Source: CAD feature listing. Evaluate the final solid. Frame: model axes, mm. Round coordinates to 2 decimals unless told otherwise and drop trailing zeros. Loops run counter-clockwise (first coordinate to the right, second up) from the corner with the lowest first, then second, coordinate; pieces in that order, holes last. Notation, with made-up numbers: (19.25, 5) -> (35.25, 5) arc R6 cw to (35.25, 15) -> close; hole circle Ø2 at (-31.75, 67). An arc over 180 degrees is marked (long way). Put each result on its own line as item: value. Start each with the question number.
1. Contact query for flat-ended pins moving along their axis: pin 1 (1.6 mm diameter, centred on x = -2, z = 1.5, fed in from +Y); pin 2 (2.5 mm diameter, centred on x = 13, y = -37.25, fed in from -Z); pin 3 (1 mm diameter, centred on y = -40.5, z = 0.5, fed in from +X); pin 4 (1.2 mm diameter, centred on x = -13, y = 37.25, fed in from -Z). Output: stop coordinate, or through.
2. Cut plane A-A (y = 19.5). Return the cut outline in (x, z), then the cut area to 3 significant figures.
3. Material intervals for L1, parallel to Y at x = -2.5, z = 1.2; L2, parallel to Y at x = -1, z = 0.05; L3, parallel to X at y = 10, z = 0.6, sorted ascending.
4. Cut plane D-D (y = -37.25). Return the cut outline in (x, z), then the cut area to 3 significant figures.
5. Cut plane C-C (x = -13). Return the cut outline in (y, z), then the cut area to 3 significant figures.
6. Cut plane B-B (z = 1.25). Return the cut outline in (x, y), then the cut area to 3 significant figures.
```python
from build123d import *

# Parameters (mm, degrees)
F1_DEPTH = 2
F2_R     = 1
F3_DEPTH = 2.001
F4_W     = 11.5
F4_H     = 56.5
F4_H_2   = 6.5
F5_DEPTH = 2.001
F6_W     = 15
F6_H     = 15
F7_DEPTH = 3
F8_SIZE  = 2


with BuildPart() as f1:
    # F0 (on Top) → F1 (new body)
    with BuildSketch(Plane.XY):
        with BuildLine():
            Line((16.75, -33), (16.75, 33))
            ThreePointArc((16.75, 33), (11.844039, 44.844039), (0, 49.75))
            ThreePointArc((0, 49.75), (-11.844039, 44.844039), (-16.75, 33))
            Line((-16.75, 33), (-16.75, -33))
            ThreePointArc((-16.75, -33), (-11.844039, -44.844039), (0, -49.75))
            ThreePointArc((0, -49.75), (11.844039, -44.844039), (16.75, -33))
        make_face()
    extrude(amount=F1_DEPTH)

    # F2 (on face) → F3 (cut, through all)
    with BuildSketch(Plane.XY.offset(2)):
        with Locations((-13, -37.25)):
            Circle(F2_R)
        with Locations((13, -37.25)):
            Circle(F2_R)
        with Locations((13, 37.25)):
            Circle(F2_R)
        with Locations((-13, 37.25)):
            Circle(F2_R)
    extrude(amount=-F3_DEPTH, mode=Mode.SUBTRACT)

    # F4 (on face) → F5 (cut, through all)
    with BuildSketch(Plane.XY.offset(2)):
        with Locations((0, 16.25)):
            Rectangle(F4_W, F4_H)
        with Locations((0, -41.75)):
            Rectangle(F4_W, F4_H_2)
    extrude(amount=-F5_DEPTH, mode=Mode.SUBTRACT)

    # F6 (on face) → F7 (join)
    with BuildSketch(Plane(origin=(0, 0, 0), x_dir=(1, 0, 0), z_dir=(0, 0, -1))):
        with Locations((0, 26)):
            Rectangle(F6_W, F6_H)
    extrude(amount=F7_DEPTH)

    # F8
    f8_edges = [f1.edges().sort_by_distance(p)[0] for p in [
        (0, -33.5, -3),
        (-7.5, -26, -3),
        (0, -18.5, -3),
        (7.5, -26, -3),
    ]]
    chamfer(f8_edges, length=F8_SIZE)


solid = f1.part
```
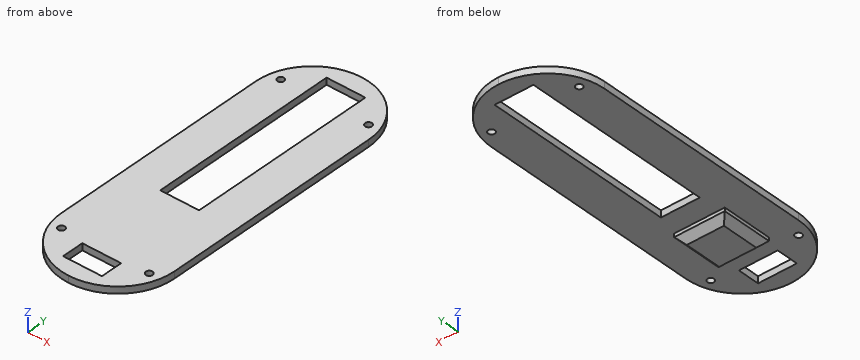
Solution:
1. pin 1: stops at y = 49.71
1. pin 2: stops at z = 0
1. pin 3: stops at x = 15.22
1. pin 4: passes through
2. outline: (-16.75, 0) -> (-5.75, 0) -> (-5.75, 2) -> (-16.75, 2) -> close; (5.75, 0) -> (16.75, 0) -> (16.75, 2) -> (5.75, 2) -> close
2. area: 44.0 mm^2
3. L1: y = -49.56 to -45, -38.5 to -12, 44.5 to 49.56
3. L2: y = -49.72 to -45, -38.5 to -12, 44.5 to 49.72
3. L3: x = -16.75 to -5.75, 5.75 to 16.75
4. outline: (-16.2, 0) -> (-14, 0) -> (-14, 2) -> (-16.2, 2) -> close; (-12, 0) -> (12, 0) -> (12, 2) -> (-12, 2) -> close; (14, 0) -> (16.2, 0) -> (16.2, 2) -> (14, 2) -> close
4. area: 56.8 mm^2
5. outline: (-43.56, 0) -> (-38.25, 0) -> (-38.25, 2) -> (-43.56, 2) -> close; (-36.25, 0) -> (36.25, 0) -> (36.25, 2) -> (-36.25, 2) -> close; (38.25, 0) -> (43.56, 0) -> (43.56, 2) -> (38.25, 2) -> close
5. area: 166 mm^2
6. outline: (-16.75, -33) arc R16.75 ccw to (0, -49.75) arc R16.75 ccw to (16.75, -33) -> (16.75, 33) arc R16.75 ccw to (0, 49.75) arc R16.75 ccw to (-16.75, 33) -> close; hole circle Ø2 at (-13, -37.25); hole circle Ø2 at (-13, 37.25); hole (-5.75, -45) -> (5.75, -45) -> (5.75, -38.5) -> (-5.75, -38.5) -> close; hole (-5.75, -12) -> (5.75, -12) -> (5.75, 44.5) -> (-5.75, 44.5) -> close; hole circle Ø2 at (13, -37.25); hole circle Ø2 at (13, 37.25)
6. area: 2,360 mm^2
